For this review, use the dimensioned drawing (mm, ordinates from the lowest corner) and the shaded views. A direction names the side the tool comes from. Give positions to 0.01 mm unless a question says otherwise; leave off trailing zeros. Order: outer loops, then holes, each group sorted by start corner. A loop starts at its lowest first (then second) coordinate and runs counter-clockwise, first axis right, second up. Notation, with made-up numbers: (88.5, 74.5) - (126.5, 74.5) arc R10 ccw to (126.5, 79.5) - close; hole circle Ø8 at (-2.75, 82.5). An arc over 180 degrees is marked (long way). Use a Markdown table: item, result. Add a question column.
1) Clearance check with flat-ended pins moving along their axes: P1, Ø5, axis at x = 67, z = 19.5, coming from the -Y side; P2, Ø6, axis at x = 77.5, y = 38.72, coming from the +Z side; P3, Ø5, axis at y = 13.5, z = 10.5, coming from the +X side. State where each tip first meets the part, or that it passes through.
2) We need section A-A on z = 7.25. Write out the cut boundary in (x, y) (1 decimal), then the cut area to 3 significant figures.
3) Machinability: for the marked faces 4 and 5, which of the approach directions +Z, -Z, +X, -X, +Y, -Y give a long, thin tool a straight path to every point of the face, cutting with its end or side? Answer none if there is none.
4) We need section D-D on x = 75.5. Write out the cut boundary in (y, z) (1 decimal), then the cut area to 3 significant figures.
5) Mouldability with a two-part tool opening along Y and no side actions: class the marked faces 1, 2 and 3 as released by +Y, released by -Y, zero draft, split by the parting line, or undercut.
6) We need section C-C on z = 21.5. Write out the cut boundary in (x, y) (1 decimal), then the cut area to 3 significant figures.
7) Wall thickness on L1, parallel to Y at x = 32.5, z = 19.5 (1 decimal); L2, parallel to X at y = 6.5, z = 15.5 (1 decimal); L3, parallel to Y at x = 30.5, z = 19.5 (1 decimal): over which ranges is each line inside the solid? List them lowest first.
8) We need section B-B on y = 6. Write out the cut boundary in (x, z).
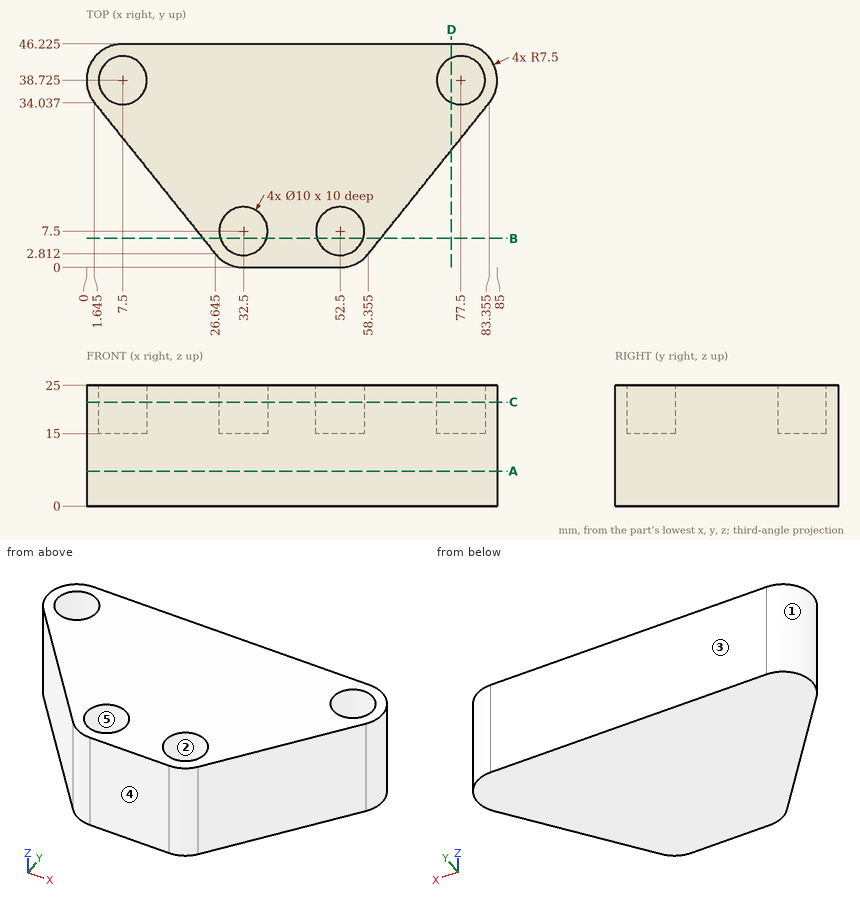
Checked values:
| question | item | result |
|---|---|---|
| 1 | P1 | y = 10.49 |
| 1 | P2 | z = 15 |
| 1 | P3 | x = 68.91 |
| 2 | outline | (1.6, 34) - (26.6, 2.8) arc R7.5 ccw to (32.5, 0) - (52.5, 0) arc R7.5 ccw to (58.4, 2.8) - (83.4, 34) arc R7.5 ccw to (77.5, 46.2) - (7.5, 46.2) arc R7.5 ccw to start |
| 2 | area | 2,860 mm² |
| 3 | face 4 | +Z, -Z, +X, -X, -Y |
| 3 | face 5 | +Z |
| 4 | outline | (24.2, 0) - (46.2, 0) - (46.2, 25) - (43.3, 25) - (43.3, 15) - (34.1, 15) - (34.1, 25) - (24.2, 25) - close |
| 4 | area | 458 mm² |
| 5 | face 1 | split by the parting line |
| 5 | face 2 | undercut |
| 5 | face 3 | released by +Y |
| 6 | outline | (1.6, 34) - (26.6, 2.8) arc R7.5 ccw to (32.5, 0) - (52.5, 0) arc R7.5 ccw to (58.4, 2.8) - (83.4, 34) arc R7.5 ccw to (77.5, 46.2) - (7.5, 46.2) arc R7.5 ccw to start; hole circle Ø10 at (7.5, 38.7); hole circle Ø10 at (32.5, 7.5); hole circle Ø10 at (52.5, 7.5); hole circle Ø10 at (77.5, 38.7) |
| 6 | area | 2,540 mm² |
| 7 | L1 | 0 to 2.5, 12.5 to 46.2 |
| 7 | L2 | 23.7 to 27.6, 37.4 to 47.6, 57.4 to 61.3 |
| 7 | L3 | 0.3 to 2.9, 12.1 to 46.2 |
| 8 | outline | (24.09, 0) - (60.91, 0) - (60.91, 25) - (57.27, 25) - (57.27, 15) - (47.73, 15) - (47.73, 25) - (37.27, 25) - (37.27, 15) - (27.73, 15) - (27.73, 25) - (24.09, 25) - close |
